The listing builds one solid part. Answer for the finished solid, in the listing's coordinates (mm). Face numbers are marked on the shaded views. Coordinates: 2 decimals unless noted, no trailing zeros. Order: outer loops, then holes, each group sorted by start corner. A loop starts at its lowest first (then second) coordinate and runs counter-clockwise, first axis right, second up. Notation, with made-up numbers: (44.25, -7.5) -> (48.25, -7.5) arc R19 ccw to (48.25, -2.5) -> close; hole circle Ø2 at (74.25, -9). An arc over 180 degrees is marked (long way). One line per question, with ' | ' between items.
from build123d import *

# Parameters (mm, degrees)
SKETCH_1_W             = 165
SKETCH_1_H             = 50
SM_BASE_FLANGE_1_DEPTH = 1
SM_EDGE_FLANGE_1_DEPTH = 50
SKETCH_9_R             = 18.474720046
CUT_EXTRUDE_1_DEPTH    = 10
SM_EDGE_FLANGE_2_DEPTH = 165


# Sheet-metal steps are written as plain solids
with BuildPart() as part:
    # Sketch 1 → 基体-法兰1 (new body)
    with BuildSketch(Plane(origin=(0, 0, 0), x_dir=(1, 0, 0), z_dir=(0, 1, 0))):
        Rectangle(SKETCH_1_W, SKETCH_1_H)
    extrude(amount=-SM_BASE_FLANGE_1_DEPTH)

    # 边线-法兰1 section (across the edge) → 边线-法兰1 (add)
    with BuildSketch(Plane(origin=(-82.6, 0, -25), x_dir=(1, 0, 0), z_dir=(0, 0, 1))):
        with BuildLine():
            Line((-1, 0.1), (-1, 49))
            Line((-1, 49), (0, 49))
            Line((0, 49), (0, 0.1))
            ThreePointArc((0, 0.1), (0.029289322, 0.029289322), (0.1, 0))
            Line((0.1, 0), (0.1, -1))
            ThreePointArc((0.1, -1), (-0.677817459, -0.677817459), (-1, 0.1))
        make_face()
    sm_edge_flange_1 = extrude(amount=SM_EDGE_FLANGE_1_DEPTH)

    # 镜向1: 边线-法兰1 across plane
    add(sm_edge_flange_1.mirror(Plane(origin=(0, 0, 0), x_dir=(0, 0, 1), z_dir=(1, 0, 0))))

    # 草图9 → 切除-拉伸1 (cut)
    with BuildSketch(Plane(origin=(0, 0, 0), x_dir=(1, 0, 0), z_dir=(0, 1, 0))):
        with Locations((0, -25)):
            Circle(SKETCH_9_R)
    extrude(amount=-CUT_EXTRUDE_1_DEPTH, mode=Mode.SUBTRACT)

    # 边线-法兰2 section (across the edge) → 边线-法兰2 (add)
    with BuildSketch(Plane(origin=(82.5, 0, -25.041421356), x_dir=(0, 0.7071067811865512, 0.7071067811865438), z_dir=(-1, 0, 0))):
        with BuildLine():
            Line((-1, 0.041421356), (-1, 34.585786438))
            Line((-1, 34.585786438), (0, 34.585786438))
            Line((0, 34.585786438), (0, 0.041421356))
            ThreePointArc((0, 0.041421356), (0.007612047, 0.003153013), (0.029289322, -0.029289322))
            Line((0.029289322, -0.029289322), (-0.677817459, -0.736396103))
            ThreePointArc((-0.677817459, -0.736396103), (-0.916267486, -0.379530419), (-1, 0.041421356))
        make_face()
    extrude(amount=SM_EDGE_FLANGE_2_DEPTH)


solid = part.part
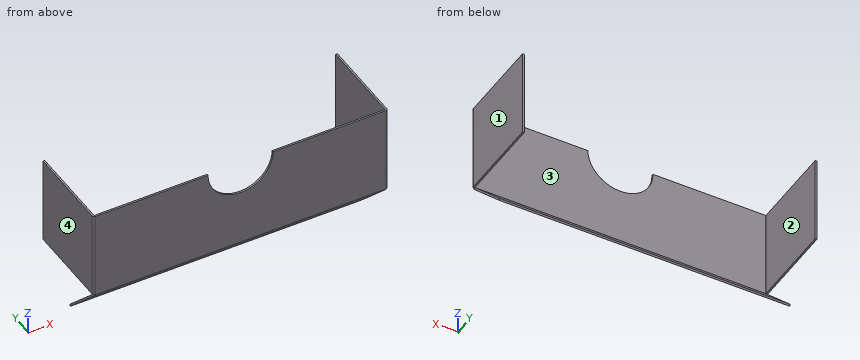
Item 1: Determine the mould class of the marked faces 1, 2, 3 and 4 for opening direction X: pulls with the +X half, pulls with the -X half, needs draft (parallel to the pull), parting line crosses it, or undercut.
Computed values:
face 1: pulls with the +X half | face 2: undercut | face 3: undercut | face 4: pulls with the -X half
Item 2: Each of these flat-tipped pins is pushed along its axis until it touches: pin 1 Ø5 at (x, z) = (-41.5, -41.5) entering from +Y; pin 2 Ø5 at (y, z) = (33, -26) entering from -X; pin 3 Ø6 at (x, z) = (1.5, -38.5) entering from -Y; pin 4 Ø7.5 at (y, z) = (10, -41) entering from -X. Where does it stop, or does it pass through?
Computed values:
pin 1: stops at y = 18.96 | pin 2: stops at x = -83.6 | pin 3: stops at y = 9.04 | pin 4: stops at x = -82.5
Item 3: Section A-A, the plane y = 46 is taken. Give the vertices of the cut face in (x, z), plus the area to 3 significant figures.
Computed values:
outline: (-83.6, -25) -> (-82.6, -25) -> (-82.6, 25) -> (-83.6, 25) -> close; (82.6, -25) -> (83.6, -25) -> (83.6, 25) -> (82.6, 25) -> close | area: 100 mm^2
Item 4: Section B-B, the plane x = -66.5 is taken. Give the vertices of the cut face in (y, z).
Computed values:
outline: (-1, -25) arc R1.1 ccw to (-0.68, -25.78) -> (23.75, -50.2) -> (24.46, -49.5) -> (0.03, -25.07) arc R0.1 cw to (0, -25) -> (0, 25) -> (-1, 25) -> close
Item 5: Section D-D, the plane y = 8.5 is taken. Give the vertices of the cut face in (x, z), plus the area to 3 significant figures.
Computed values:
outline: (-83.6, -25) -> (-82.6, -25) -> (-82.6, 25) -> (-83.6, 25) -> close; (-82.5, -34.96) -> (82.5, -34.96) -> (82.5, -33.54) -> (-82.5, -33.54) -> close; (82.6, -25) -> (83.6, -25) -> (83.6, 25) -> (82.6, 25) -> close | area: 333 mm^2
Item 6: Section C-C, the plane z = -3 is taken. Give the vertices of the cut face in (x, y).
Computed values:
outline: (-83.6, 0.1) arc R1.1 ccw to (-82.5, -1) -> (82.5, -1) arc R1.1 ccw to (83.6, 0.1) -> (83.6, 49) -> (82.6, 49) -> (82.6, 0.1) arc R0.1 cw to (82.5, 0) -> (-82.5, 0) arc R0.1 cw to (-82.6, 0.1) -> (-82.6, 49) -> (-83.6, 49) -> close
Item 7: Find the intervals of material crossed by L1, parallel to X at y = 18.5, z = 12.5; L2, parallel to Y at x = 67, z = -13; L3, parallel to Z at x = 73.5, y = 22, in increasing order.
Computed values:
L1: x = -83.6 to -82.6, 82.6 to 83.6 | L2: y = -1 to 0 | L3: z = -48.46 to -47.04
